Autodesk Inventor part; units mm, degrees
ref_plane "YZ Plane" through (0, 0, 0) normal (1, 0, 0) x (0, 1, 0)
ref_plane "XZ Plane" through (0, 0, 0) normal (0, 1, 0) x (-1, 0, 0)
ref_plane "XY Plane" through (0, 0, 0) normal (0, 0, 1) x (1, 0, 0)
sketch "Эскиз1" plane through (0, 0, 0) normal (0, 0, 1) x (1, 0, 0)
  line L0 (-7, -3.5) -> (7, -3.5) construction
  line L1 (7, -3.5) -> (7, 3.5)
  line L2 (7, 3.5) -> (-7, 3.5)
  line L3 (-7, 3.5) -> (-7, -3.5)
  line L4 (-7, -3.5) -> (7, 3.5) construction
  line L5 (7, -3.5) -> (-7, 3.5) construction
  line L6 (0, -3.5) -> (0, -12.5) construction
  line L7 (-7, -3.5) -> (-3.289, -13.697)
  line L8 (7, -3.5) -> (3.289, -13.697)
  arc A0 (-3.289, -13.697) -> (3.289, -13.697) centre (0, -12.5) ccw
  point P0 (0, 0)
  point P1 (0, 0)
  point P2 (0, 0)
  point P3 (0, 0)
  dimension "d0" = 14
  dimension "d1" = 7
  dimension "d4" = 9
  dimension "d5" = 3.5
extrude "Выдавливание1" add sketch "Эскиз1" along normal blind 1.5
sketch "Эскиз2" plane through (0, 0, 1.5) normal (0, 0, 1) x (1, 0, 0)
  arc A0 (-3.289, -13.697) -> (3.289, -13.697) centre (0, -12.5) ccw construction
  circle A1 centre (0, -12.5) radius 2.5
  circle A2 centre (0, -12.5) radius 1.5
  point P0 (0, 0)
  dimension "d8" = 5
  dimension "d39" = 1
extrude "Выдавливание11" add sketch "Эскиз2" along normal blind 5
fillet "Сопряжение1" radius 3.5 2 edges at (7, 3.5, 0.75) (-7, 3.5, 0.75)
sketch "Эскиз5" plane through (0, 0, 0) normal (0, 0, 1) x (1, 0, 0)
  circle A0 centre (0, -12.5) radius 1.25 construction
  line L0 (0, -3.5) -> (0, 3.5) construction
  circle A1 centre (3.5, 0) radius 0.5
  line L1 (3.5, 0) -> (3.5, 3.5) construction
  line L2 (3.5, 0) -> (0, 0) construction
  line L3 (7, 3.5) -> (-7, 3.5) construction
  circle A2 centre (-3.5, 0) radius 0.5
  point P0 (7, -3.5)
  dimension "d34" = 1
  dimension "d35" = 3.5
hole "Отверстие1" at (-3.5, 0, 0) at (3.5, 0, 0) direction (0, 0, 1) diameter 1 end through all countersink diameter 1.5 countersink angle 90
properties part number "переходник2"
Source: CAD feature listing. Evaluate the final solid. Frame: model axes, mm. A direction names the side the tool comes from. Round coordinates to 2 decimals unless told otherwise and drop trailing zeros. Loops run counter-clockwise (first coordinate to the right, second up) from the corner with the lowest first, then second, coordinate; pieces in that order, holes last. Notation, with made-up numbers: M -34,60 L -16,60 A11 cw -16,67 Z; hole C -38,13 d9. An arc over 180 degrees is marked long. Return JSON: item names as keys, results as strings. Group by question number.
1. Material intervals for line 1 along X through (y, z) = (0, 1.2); line 2 along Z through (x, y) = (-1, 0); line 3 along Y through (x, z) = (0, 3.5), sorted ascending. Write a range as from..to.
2. Section query C-C on y = -11.5. Output: boundary loops of the cut face in (x, z), and give its area (3 significant figures).
3. Section query A-A on x = 0. Output: boundary loops of the cut face in (y, z).
4. Reachability of faces 4 (the face through (0, -11, 4)), 5 (the face through (-4, 0, 1)) from +Z, -Z, +X, -X, +Y, -Y: full face, straight path, thin tool, end or side. Return the list, or none.
5. Section query B-B on z = 6. Output: boundary loops of the cut face in (x, y).
6. Pin query (flat end, axial travel): pin 1 (3 mm diameter, centred on x = -4, y = -6, fed in from +Z); pin 2 (1.5 mm diameter, centred on y = -10, z = 2, fed in from +X); pin 3 (1.5 mm diameter, centred on x = 0, z = 3, fed in from -Y). Return the tip coordinate at first contact, or that it passes through.
7. Section query D-D on y = -1. Output: boundary loops of the cut face in (x, z).
8. Mould query, pull axis X, two halves, no side actions, for faces 1 (the face through (0, -12, 1.5)), 2 (the face through (7, -2, 1)), 3 (the face through (-5, -9, 1)). Classes: released by +X, released by -X, zero draft, split by the parting line, or undercut.
Checks:
{
 "1": {"line 1": "x = -7..-4, -3..3, 4..7", "line 2": "z = 0..1.5", "line 3": "y = -15..-14, -11..-10"},
 "2": {"outline": "M -4.09,0 L 4.09,0 L 4.09,1.5 L 2.29,1.5 L 2.29,6.5 L 1.12,6.5 L 1.12,1.5 L -1.12,1.5 L -1.12,6.5 L -2.29,6.5 L -2.29,1.5 L -4.09,1.5 Z", "area": "24.0 mm²"},
 "3": {"outline": "M -16,0 L 3.5,0 L 3.5,1.5 L -10,1.5 L -10,6.5 L -11,6.5 L -11,1.5 L -14,1.5 L -14,6.5 L -15,6.5 L -15,1.5 L -16,1.5 Z"},
 "4": {"face 4": "+Z", "face 5": "+Z, -Z"},
 "5": {"outline": "C 0,-12.5 d5; hole C 0,-12.5 d3"},
 "6": {"pin 1": "stops at z = 1.5", "pin 2": "stops at x = 4.84", "pin 3": "stops at y = -15"},
 "7": {"outline": "M -7,0 L 7,0 L 7,1.5 L -7,1.5 Z"},
 "8": {"face 1": "undercut", "face 2": "released by +X", "face 3": "released by -X"}
}
